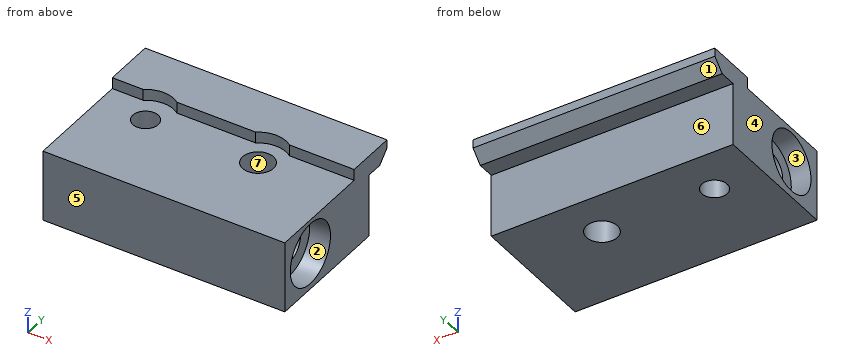
from build123d import *

# Parameters (mm, degrees)
F0_W      = 43
F0_H      = 23
F1_DEPTH  = 12.7
F2_R      = 2.75
F2_R_2    = 2.25
F3_DEPTH  = 25.4
F4_R      = 3
F5_DEPTH  = 50.8
F6_R      = 5.35
F7_DEPTH  = 3.5
F8_R      = 5.5
F9_DEPTH  = 3.7
F10_W     = 43
F10_H     = 4
F11_DEPTH = 2
F12_W     = 43
F12_H     = 3.5
F13_DEPTH = 5
F14_SIZE  = 2
F15_R     = 5
F16_DEPTH = 25


with BuildPart() as f1:
    # F0 (on Top) → F1 (new body)
    with BuildSketch(Plane.XY):
        Rectangle(F0_W, F0_H)
    extrude(amount=F1_DEPTH)

    # F2 (on face) → F3 (cut)
    with BuildSketch(Plane.XY.offset(12.7)):
        with Locations((7, 3.5)):
            Circle(F2_R)
        with Locations((-13, 3.5)):
            Circle(F2_R_2)
    extrude(amount=-F3_DEPTH, mode=Mode.SUBTRACT)

    # F4 (on face) → F5 (cut)
    with BuildSketch(Plane(origin=(-21.5, 0, 0), x_dir=(0, -1, 0), z_dir=(-1, 0, 0))):
        with Locations((4.5, 6.5)):
            Circle(F4_R)
    extrude(amount=-F5_DEPTH, mode=Mode.SUBTRACT)

    # F6 (on face) → F7 (cut)
    with BuildSketch(Plane(origin=(-21.5, 0, 0), x_dir=(0, -1, 0), z_dir=(-1, 0, 0))):
        with Locations((4.5, 6.5)):
            Circle(F6_R)
    extrude(amount=-F7_DEPTH, mode=Mode.SUBTRACT)

    # F8 (on face) → F9 (cut)
    with BuildSketch(Plane.YZ.offset(21.5)):
        with Locations((-4.5, 6.5)):
            Circle(F8_R)
    extrude(amount=-F9_DEPTH, mode=Mode.SUBTRACT)

    # F10 (on face) → F11 (join)
    with BuildSketch(Plane.XY.offset(12.7)):
        with Locations((0, 9.5)):
            Rectangle(F10_W, F10_H)
    extrude(amount=F11_DEPTH)

    # F12 (on face) → F13 (join)
    with BuildSketch(Plane(origin=(0, 11.5, 0), x_dir=(-1, 0, 0), z_dir=(0, 1, 0))):
        with Locations((0, 12.95)):
            Rectangle(F12_W, F12_H)
    extrude(amount=F13_DEPTH)

    # F14
    f14_edges = [f1.edges().sort_by_distance(p)[0] for p in [
        (0, 16.5, 11.2),
    ]]
    chamfer(f14_edges, length=F14_SIZE)

    # F15 (on face) → F16 (cut)
    with BuildSketch(Plane.XY.offset(12.7)):
        with Locations((-13, 3.5)):
            Circle(F15_R)
        with Locations((7, 3.5)):
            Circle(F15_R)
    extrude(amount=F16_DEPTH, mode=Mode.SUBTRACT)


solid = f1.part
Geometry check sheet. Reference: the model listing, model coordinates, mm. Face numbers are marked on the shaded views. A direction names the side the tool comes from. Give positions to 0.01 mm unless a question says otherwise; leave off trailing zeros. Loops run counter-clockwise (first coordinate to the right, second up) from the corner with the lowest first, then second, coordinate; pieces in that order, holes last. Notation, with made-up numbers: M -13,81 L 11,81 A30 cw 11,117 Z; hole C 61.5,-23.5 d6. An arc over 180 degrees is marked long. Answer as a JSON object with one key per item and string values. Group by question number.
Item 1: Access from +Z, -Z, +X, -X, +Y, -Y to the whole of each face (thin tool, end or side, straight path). Record for the marked faces 1, 2 and 3.
Item 2: Sectioned sample at D-D on z = 5.5. Record the boundary of the cut face in (x, y).
Item 3: Sectioned sample at B-B on y = 2. Record the boundary of the cut face in (x, z).
Item 4: Sectioned sample at C-C on x = 2. Record the boundary of the cut face in (y, z), plus the area to 3 significant figures.
Item 5: Sectioned sample at A-A on x = 7. Record the boundary of the cut face in (y, z).
Item 6: Gauge pin test, flat ends, axial feed: pin 1 (0.9 mm diameter, centred on x = 0, y = 12.5, fed in from -Z); pin 2 (8 mm diameter, centred on x = 1.5, z = 4.5, fed in from +Y); pin 3 (6.5 mm diameter, centred on y = -4.5, z = 6.5, fed in from +X); pin 4 (1 mm diameter, centred on y = 13, z = 5.5, fed in from -X). Record the tip position at first contact, or that the pin passes through.
Item 7: Mould release check, pull along Y, two halves, no side actions. Record for the marked faces 4, 5, 6 and 7: pulls with the +Y half, pulls with the -Y half, needs draft (parallel to the pull), parting line crosses it, or undercut.
Item 8: Material ranges on L1, parallel to Z at x = -7, y = -4.5; L2, parallel to Z at x = -6, y = -1.25; L3, parallel to X at y = -3, z = 1.5, recorded low to high.
Findings below:
{
 "1": {"face 1": "-Z, +X, -X, +Y", "face 2": "+X", "face 3": "-X"},
 "2": {"outline": "M -21.5,-11.5 L 21.5,-11.5 L 21.5,-9.91 L 17.8,-9.91 L 17.8,-7.33 L -18,-7.33 L -18,-9.76 L -21.5,-9.76 Z; M -21.5,0.76 L -18,0.76 L -18,-1.67 L 17.8,-1.67 L 17.8,0.91 L 21.5,0.91 L 21.5,11.5 L -21.5,11.5 Z; hole C -13,3.5 d4.5; hole C 7,3.5 d5.5"},
 "3": {"outline": "M -21.5,0 L -14.68,0 L -14.68,12.7 L -21.5,12.7 Z; M -11.32,0 L 4.7,0 L 4.7,12.7 L -11.32,12.7 Z; M 9.3,0 L 21.5,0 L 21.5,12.7 L 9.3,12.7 Z"},
 "4": {"outline": "M -11.5,0 L 11.5,0 L 11.5,11.2 L 14.5,11.2 L 16.5,13.2 L 16.5,14.7 L 7.5,14.7 L 7.5,12.7 L -11.5,12.7 Z; hole C -4.5,6.5 d6", "area": "287 mm2"},
 "5": {"outline": "M -11.5,0 L 0.75,0 L 0.75,12.7 L -11.5,12.7 Z; M 6.25,0 L 11.5,0 L 11.5,11.2 L 14.5,11.2 L 16.5,13.2 L 16.5,14.7 L 8.5,14.7 L 8.5,12.7 L 6.25,12.7 Z; hole C -4.5,6.5 d6"},
 "6": {"pin 1": "z = 11.2", "pin 2": "y = 11.5", "pin 3": "x = 17.8", "pin 4": "through"},
 "7": {"face 4": "needs draft", "face 5": "pulls with the -Y half", "face 6": "pulls with the +Y half", "face 7": "undercut"},
 "8": {"L1": "0 to 3.5, 9.5 to 12.7", "L2": "0 to 12.7", "L3": "-18 to 17.8"}
}
